```python
from build123d import *

# Parameters (mm, degrees)
SKETCH_1_W          = 150
SKETCH_1_H          = 31
EXTRUDE_1_DEPTH     = 97
SKETCH_2_R          = 2.25
CUT_EXTRUDE_1_DEPTH = 127.471340627
SKETCH_3_W          = 10
SKETCH_3_H          = 92
CUT_EXTRUDE_2_DEPTH = 26
CUT_EXTRUDE_3_DEPTH = 5


with BuildPart() as part:
    # 草图1 → 凸台-拉伸1 (new body)
    with BuildSketch(Plane(origin=(0, 0, 0), x_dir=(1, 0, 0), z_dir=(0, 1, 0))):
        Rectangle(SKETCH_1_W, SKETCH_1_H)
    extrude(amount=EXTRUDE_1_DEPTH)

    # 草图2 → 切除-拉伸1 (cut, through all)
    with BuildSketch(Plane.XY.offset(15.5)):
        with Locations((70, 13.25)):
            Circle(SKETCH_2_R)
        with Locations((70, 78.75)):
            Circle(SKETCH_2_R)
        with BuildLine():
            Line((-75, 15.5), (-72, 15.5))
            ThreePointArc((-72, 15.5), (-69.65, 13.15), (-72, 10.8))
            Line((-72, 10.8), (-75, 10.8))
            ThreePointArc((-75, 10.8), (-77.35, 13.15), (-75, 15.5))
        make_face()
        with BuildLine():
            Line((-75, 81.2), (-72, 81.2))
            ThreePointArc((-72, 81.2), (-69.65, 78.85), (-72, 76.5))
            Line((-72, 76.5), (-75, 76.5))
            ThreePointArc((-75, 76.5), (-77.35, 78.85), (-75, 81.2))
        make_face()
    extrude(amount=-CUT_EXTRUDE_1_DEPTH, mode=Mode.SUBTRACT)

    # 草图3 → 切除-拉伸2 (cut)
    with BuildSketch(Plane.XY.offset(15.5)):
        with Locations((-70, 46)):
            Rectangle(SKETCH_3_W, SKETCH_3_H)
    cut_extrude_2 = extrude(amount=-CUT_EXTRUDE_2_DEPTH, mode=Mode.SUBTRACT)

    # 镜向1: 切除-拉伸2 across plane
    add(cut_extrude_2.mirror(Plane(origin=(0, 0, 0), x_dir=(0, 0, 1), z_dir=(1, 0, 0))), mode=Mode.SUBTRACT)

    # 草图4 → 切除-拉伸3 (cut)
    with BuildSketch(Plane.XZ.offset(-92)):
        with BuildLine():
            Line((-75, 4.85), (-72, 4.85))
            ThreePointArc((-72, 4.85), (-69.65, 2.5), (-72, 0.15))
            Line((-72, 0.15), (-75, 0.15))
            ThreePointArc((-75, 0.15), (-77.35, 2.5), (-75, 4.85))
        make_face()
    cut_extrude_3 = extrude(amount=-CUT_EXTRUDE_3_DEPTH, mode=Mode.SUBTRACT)

    # 镜向2: 切除-拉伸3 across plane
    add(cut_extrude_3.mirror(Plane(origin=(0, 0, 0), x_dir=(0, 0, 1), z_dir=(1, 0, 0))), mode=Mode.SUBTRACT)


solid = part.part
```
Can you work these out from the model? Positions are in its coordinate system, mm. A direction names the side the tool comes from. Give positions to 0.01 mm unless a question says otherwise; leave off trailing zeros. Loops run counter-clockwise (first coordinate to the right, second up) from the corner with the lowest first, then second, coordinate; pieces in that order, holes last. Notation, with made-up numbers: M 3.5,80 L 33.5,80 A37 cw 33.5,116 Z; hole C 59.5,62 d1. An arc over 180 degrees is marked long. One line per question, with ' | ' between items. Start each with the question number.
Q1. If we section it at C-C (y = 13.25): Please give me the cut outline in (x, z), plus the area to 3 significant figures.
Q2. For pin 1 Ø10 at (y, z) = (54, 3.5) entering from -X; pin 2 Ø1 at (y, z) = (68, 10.5) entering from +X; pin 3 Ø3 at (x, y) = (72, 65.5) entering from +Z, each with a flat end and sliding along its axis, tell me the tip position at first contact or that it passes through.
Q3. If I drill on line 1 (Y direction, x = 70, z = -13.65); line 2 (X direction, y = 13, z = -14); line 3 (X direction, y = 85.5, z = 7.5), over which ranges is the centre line in solid material (lowest first)? Write a range as from..to.
Q4. For faces 4 (the flat face through (-70, 47, -10.5)), 5 (the flat face through (-74, 15.5, -13)), 6 (the flat face through (-73, 94, 0.15)), which set-ups out of +Z, -Z, +X, -X, +Y, -Y let a thin tool reach every point of the face, with its end or its side?
Q5. If we mould it in two halves opening along Z, with no side actions, what happens to faces 1 (the flat face through (-75, 46, -13)), 2 (the flat face through (73, 94, 0.15)), 3 (the flat face through (-1, 48, 15.5))? For each: +Z half, -Z half, draft (parallel to the pull), parting line (faces both ways), or undercut.
Q6. If we section it at B-B (z = 2.5): Please give me the cut outline in (x, y), plus the area to 3 significant figures.
Q7. If we section it at A-A (y = 84): Please give me the cut outline in (x, z), plus the area to 3 significant figures.
Computed:
1) outline: M -69.65,-15.5 L 67.75,-15.5 L 67.75,-10.5 L 65,-10.5 L 65,15.5 L -65,15.5 L -65,-10.5 L -69.65,-10.5 Z; M 72.25,-15.5 L 75,-15.5 L 75,-10.5 L 72.25,-10.5 Z | area: 4,080 mm²
2) pin 1: stops at x = -65 | pin 2: stops at x = 65 | pin 3: stops at z = -10.5
3) line 1: y = 0..11, 15.5..76.5, 81..97 | line 2: x = -69.65..67.76, 72.24..75 | line 3: x = -65..65
4) face 4: +Z, -X, -Y | face 5: +Z, -Z, -X | face 6: -X, +Y, -Y
5) face 1: draft | face 2: undercut | face 3: +Z half
6) outline: M -69.65,92 L -65,92 L -65,0 L 65,0 L 65,92 L 69.65,92 L 69.65,97 L -69.65,97 Z | area: 12,700 mm²
7) outline: M -75,-15.5 L 75,-15.5 L 75,-10.5 L 65,-10.5 L 65,15.5 L -65,15.5 L -65,-10.5 L -75,-10.5 Z | area: 4,130 mm²
